The figure shows three views and two pictorial views of one solid part (mm, origin at its lowest corner). Answer the questions. A direction names the side the tool comes from. Coordinates: 2 decimals unless noted, no trailing zeros. Loops run counter-clockwise (first coordinate to the right, second up) from the corner with the lowest first, then second, coordinate; pieces in that order, holes last. Notation, with made-up numbers: (16.25, 8) -> (65.25, 8) arc R13 ccw to (65.25, 25) -> close; hole circle Ø2 at (71, 8.25). An arc over 180 degrees is marked (long way). Answer as a JSON object with one key per item and string values. Group by question number.
1) Section B-B, the plane y = 120.65 is taken. Give the vertices of the cut face in (x, z).
2) Flat-ended cylindrical pins translate along their axes: P1, Ø8, axis at y = 45, z = 10.5, coming from the +X side (3 decimals); P2, Ø1, axis at y = 60, z = 33.5, coming from the -X side (3 decimals); P3, Ø9.5, axis at x = 12, y = 40, coming from the -Z side (3 decimals). Find the tip coordinate at first contact, or state that the pin passes through.
3) Section D-D, the plane z = 40 is taken. Give the vertices of the cut face in (x, y) (1 decimal), plus the area to 3 significant figures.
4) Which of the six approach directions +Z, -Z, +X, -X, +Y, -Y give full straight-line access (tool end or side, diameter ignored) to the marked faces 1, 2 and 3?
5) Determine the mould class of the marked faces 4, 5 and 6 for opening direction Y: released by +Y, released by -Y, zero draft, split by the parting line, or undercut.
6) Consider probe 1 along Y at (x, z) = (20.25, 25.4); probe 2 along X at (y, z) = (120.65, 4); probe 3 along Y at (x, z) = (12.7, 8.75). Determine where each line is inside the solid, lowest interval first. Write a range as [from, to].
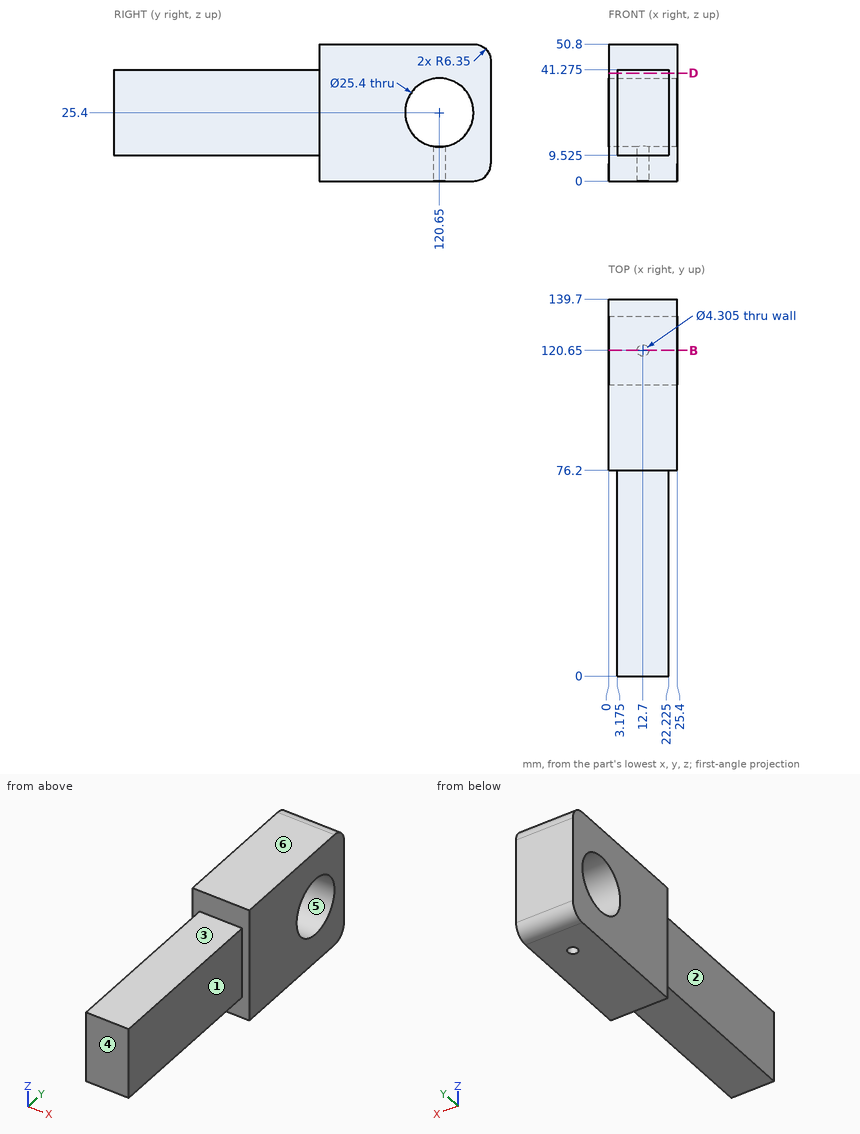
Determined:
{
 "1": {"outline": "(0, 0) -> (10.55, 0) -> (10.55, 12.7) -> (0, 12.7) -> close; (0, 38.1) -> (25.4, 38.1) -> (25.4, 50.8) -> (0, 50.8) -> close; (14.85, 0) -> (25.4, 0) -> (25.4, 12.7) -> (14.85, 12.7) -> close"},
 "2": {"P1": "x = 22.225", "P2": "x = 3.175", "P3": "z = 9.525"},
 "3": {"outline": "(0, 76.2) -> (3.2, 76.2) -> (3.2, 0) -> (22.2, 0) -> (22.2, 76.2) -> (25.4, 76.2) -> (25.4, 139.7) -> (0, 139.7) -> close", "area": "3,060 mm²"},
 "4": {"face 1": "+Z, -Z, +X, -Y", "face 2": "+Z, -Z, -X, -Y", "face 3": "+Z, +X, -X, -Y"},
 "5": {"face 4": "released by -Y", "face 5": "undercut", "face 6": "zero draft"},
 "6": {"probe 1": "[0, 107.95], [133.35, 139.7]", "probe 2": "[0, 10.55], [14.85, 25.4]", "probe 3": "[76.2, 118.5], [122.8, 139.7]"}
}
